Check sheet for the modelled part. Datum: model origin and axes. Units: mm. Round coordinates to 2 decimals unless told otherwise and drop trailing zeros. Loops run counter-clockwise (first coordinate to the right, second up) from the corner with the lowest first, then second, coordinate; pieces in that order, holes last. Notation, with made-up numbers: (-28.5, 29.25) - (27.5, 29.25) arc R16 cw to (27.5, 45.25) - close; hole circle Ø8 at (3, 10). An arc over 180 degrees is marked (long way). Put each result on its own line as item: value.
```python
from build123d import *

# Parameters (mm, degrees)
SKETCH1_W           = 89.5
SKETCH1_H           = 50.8
BOSS_EXTRUDE1_DEPTH = 1.5875
CHAMFER1_SIZE       = 2
SKETCH2_W           = 17.9768
SKETCH2_H           = 11.576
SKETCH2_W_2         = 9.4
SKETCH2_H_2         = 11.4
CUT_EXTRUDE1_DEPTH  = 2.5875
SKETCH3_R           = 1.75
CUT_EXTRUDE2_DEPTH  = 2.5875
CHAMFER2_SIZE       = 1.27
CUT_EXTRUDE3_DEPTH  = 2.5875


with BuildPart() as part:
    # Sketch1 → Boss-Extrude1 (new body)
    with BuildSketch(Plane.XY):
        with Locations((44.75, 25.4)):
            Rectangle(SKETCH1_W, SKETCH1_H)
    extrude(amount=BOSS_EXTRUDE1_DEPTH)

    # Chamfer1
    chamfer1_edges = [part.edges().sort_by_distance(p)[0] for p in [
        (0, 50.8, 0.79375),
        (89.5, 50.8, 0.79375),
        (89.5, 0, 0.79375),
        (0, 0, 0.79375),
    ]]
    chamfer(chamfer1_edges, length=CHAMFER1_SIZE)

    # Sketch2 → Cut-Extrude1 (cut, through all)
    with BuildSketch(Plane.XY.offset(1.5875)):
        with Locations((37.701291048, 34.400499876)):
            Rectangle(SKETCH2_W, SKETCH2_H)
        with Locations((62.186773048, 34.312499876)):
            Rectangle(SKETCH2_W_2, SKETCH2_H_2)
        with BuildLine():
            Line((55.722947048, 29.966053267), (55.722947048, 30.712499876))
            ThreePointArc((55.722947048, 30.712499876), (55.503277134, 31.242829962), (54.972947048, 31.462499876))
            Line((54.972947048, 31.462499876), (48.572947048, 31.462499876))
            ThreePointArc((48.572947048, 31.462499876), (48.042616962, 31.242829962), (47.822947048, 30.712499876))
            Line((47.822947048, 30.712499876), (47.822947048, 29.966053267))
            ThreePointArc((47.822947048, 29.966053267), (47.880037399, 29.679040693), (48.042616962, 29.435723181))
            Line((48.042616962, 29.435723181), (48.646170353, 28.83216979))
            ThreePointArc((48.646170353, 28.83216979), (48.889487865, 28.669590227), (49.176500439, 28.612499876))
            Line((49.176500439, 28.612499876), (54.369393658, 28.612499876))
            ThreePointArc((54.369393658, 28.612499876), (54.656406232, 28.669590227), (54.899723744, 28.83216979))
            Line((54.899723744, 28.83216979), (55.503277134, 29.435723181))
            ThreePointArc((55.503277134, 29.435723181), (55.665856698, 29.679040693), (55.722947048, 29.966053267))
        make_face()
    extrude(amount=-CUT_EXTRUDE1_DEPTH, mode=Mode.SUBTRACT)

    # Sketch3 → Cut-Extrude2 (cut, through all)
    with BuildSketch(Plane.XY.offset(1.5875)):
        with Locations((3.75, 47.15)):
            Circle(SKETCH3_R)
        with Locations((3.75, 3.65)):
            Circle(SKETCH3_R)
        with Locations((85.75, 3.65)):
            Circle(SKETCH3_R)
        with Locations((85.75, 47.15)):
            Circle(SKETCH3_R)
    extrude(amount=-CUT_EXTRUDE2_DEPTH, mode=Mode.SUBTRACT)

    # Chamfer2
    chamfer2_edges = [part.edges().sort_by_distance(p)[0] for p in [
        (2, 47.15, 1.5875),
        (2, 3.65, 1.5875),
        (84, 3.65, 1.5875),
        (84, 47.15, 1.5875),
    ]]
    chamfer(chamfer2_edges, length=CHAMFER2_SIZE)

    # Sketch4 → Cut-Extrude3 (cut, through all)
    with BuildSketch(Plane.XY.offset(1.5875)):
        with BuildLine():
            Line((71.340625, 46.99), (71.340625, 3.81))
            ThreePointArc((71.340625, 3.81), (70.15, 2.619375), (68.959375, 3.81))
            Line((68.959375, 3.81), (68.959375, 46.99))
            ThreePointArc((68.959375, 46.99), (70.15, 48.180625), (71.340625, 46.99))
        make_face()
        with BuildLine():
            Line((45.940625, 46.99), (45.940625, 43.998499876))
            ThreePointArc((45.940625, 43.998499876), (44.75, 42.807874876), (43.559375, 43.998499876))
            Line((43.559375, 43.998499876), (43.559375, 46.99))
            ThreePointArc((43.559375, 46.99), (44.75, 48.180625), (45.940625, 46.99))
        make_face()
        with BuildLine():
            Line((45.940625, 24.802499876), (45.940625, 3.81))
            ThreePointArc((45.940625, 3.81), (44.75, 2.619375), (43.559375, 3.81))
            Line((43.559375, 3.81), (43.559375, 24.802499876))
            ThreePointArc((43.559375, 24.802499876), (44.75, 25.993124876), (45.940625, 24.802499876))
        make_face()
        with BuildLine():
            Line((51.020625, 46.99), (51.020625, 43.998499876))
            ThreePointArc((51.020625, 43.998499876), (49.83, 42.807874876), (48.639375, 43.998499876))
            Line((48.639375, 43.998499876), (48.639375, 46.99))
            ThreePointArc((48.639375, 46.99), (49.83, 48.180625), (51.020625, 46.99))
        make_face()
        with BuildLine():
            Line((51.020625, 24.802499876), (51.020625, 3.81))
            ThreePointArc((51.020625, 3.81), (49.83, 2.619375), (48.639375, 3.81))
            Line((48.639375, 3.81), (48.639375, 24.802499876))
            ThreePointArc((48.639375, 24.802499876), (49.83, 25.993124876), (51.020625, 24.802499876))
        make_face()
        with BuildLine():
            Line((56.100625, 46.99), (56.100625, 43.998499876))
            ThreePointArc((56.100625, 43.998499876), (54.91, 42.807874876), (53.719375, 43.998499876))
            Line((53.719375, 43.998499876), (53.719375, 46.99))
            ThreePointArc((53.719375, 46.99), (54.91, 48.180625), (56.100625, 46.99))
        make_face()
        with BuildLine():
            Line((56.100625, 24.802499876), (56.100625, 3.81))
            ThreePointArc((56.100625, 3.81), (54.91, 2.619375), (53.719375, 3.81))
            Line((53.719375, 3.81), (53.719375, 24.802499876))
            ThreePointArc((53.719375, 24.802499876), (54.91, 25.993124876), (56.100625, 24.802499876))
        make_face()
        with BuildLine():
            Line((61.180625, 46.99), (61.180625, 43.998499876))
            ThreePointArc((61.180625, 43.998499876), (59.99, 42.807874876), (58.799375, 43.998499876))
            Line((58.799375, 43.998499876), (58.799375, 46.99))
            ThreePointArc((58.799375, 46.99), (59.99, 48.180625), (61.180625, 46.99))
        make_face()
        with BuildLine():
            Line((61.180625, 24.802499876), (61.180625, 3.81))
            ThreePointArc((61.180625, 3.81), (59.99, 2.619375), (58.799375, 3.81))
            Line((58.799375, 3.81), (58.799375, 24.802499876))
            ThreePointArc((58.799375, 24.802499876), (59.99, 25.993124876), (61.180625, 24.802499876))
        make_face()
        with BuildLine():
            Line((66.260625, 46.99), (66.260625, 43.998499876))
            ThreePointArc((66.260625, 43.998499876), (65.07, 42.807874876), (63.879375, 43.998499876))
            Line((63.879375, 43.998499876), (63.879375, 46.99))
            ThreePointArc((63.879375, 46.99), (65.07, 48.180625), (66.260625, 46.99))
        make_face()
        with BuildLine():
            Line((66.260625, 24.802499876), (66.260625, 3.81))
            ThreePointArc((66.260625, 3.81), (65.07, 2.619375), (63.879375, 3.81))
            Line((63.879375, 3.81), (63.879375, 24.802499876))
            ThreePointArc((63.879375, 24.802499876), (65.07, 25.993124876), (66.260625, 24.802499876))
        make_face()
        with BuildLine():
            Line((76.420625, 46.99), (76.420625, 3.81))
            ThreePointArc((76.420625, 3.81), (75.23, 2.619375), (74.039375, 3.81))
            Line((74.039375, 3.81), (74.039375, 46.99))
            ThreePointArc((74.039375, 46.99), (75.23, 48.180625), (76.420625, 46.99))
        make_face()
        with BuildLine():
            Line((81.500625, 46.99), (81.500625, 3.81))
            ThreePointArc((81.500625, 3.81), (80.31, 2.619375), (79.119375, 3.81))
            Line((79.119375, 3.81), (79.119375, 46.99))
            ThreePointArc((79.119375, 46.99), (80.31, 48.180625), (81.500625, 46.99))
        make_face()
        with BuildLine():
            Line((7.999375, 46.99), (7.999375, 3.81))
            ThreePointArc((7.999375, 3.81), (9.19, 2.619375), (10.380625, 3.81))
            Line((10.380625, 3.81), (10.380625, 46.99))
            ThreePointArc((10.380625, 46.99), (9.19, 48.180625), (7.999375, 46.99))
        make_face()
        with BuildLine():
            Line((13.079375, 46.99), (13.079375, 3.81))
            ThreePointArc((13.079375, 3.81), (14.27, 2.619375), (15.460625, 3.81))
            Line((15.460625, 3.81), (15.460625, 46.99))
            ThreePointArc((15.460625, 46.99), (14.27, 48.180625), (13.079375, 46.99))
        make_face()
        with BuildLine():
            Line((18.159375, 46.99), (18.159375, 3.81))
            ThreePointArc((18.159375, 3.81), (19.35, 2.619375), (20.540625, 3.81))
            Line((20.540625, 3.81), (20.540625, 46.99))
            ThreePointArc((20.540625, 46.99), (19.35, 48.180625), (18.159375, 46.99))
        make_face()
        with BuildLine():
            Line((23.239375, 46.99), (23.239375, 3.81))
            ThreePointArc((23.239375, 3.81), (24.43, 2.619375), (25.620625, 3.81))
            Line((25.620625, 3.81), (25.620625, 46.99))
            ThreePointArc((25.620625, 46.99), (24.43, 48.180625), (23.239375, 46.99))
        make_face()
        with BuildLine():
            Line((28.319375, 24.802499876), (28.319375, 3.81))
            ThreePointArc((28.319375, 3.81), (29.51, 2.619375), (30.700625, 3.81))
            Line((30.700625, 3.81), (30.700625, 24.802499876))
            ThreePointArc((30.700625, 24.802499876), (29.51, 25.993124876), (28.319375, 24.802499876))
        make_face()
        with BuildLine():
            Line((28.319375, 46.99), (28.319375, 43.998499876))
            ThreePointArc((28.319375, 43.998499876), (29.51, 42.807874876), (30.700625, 43.998499876))
            Line((30.700625, 43.998499876), (30.700625, 46.99))
            ThreePointArc((30.700625, 46.99), (29.51, 48.180625), (28.319375, 46.99))
        make_face()
        with BuildLine():
            Line((33.399375, 24.802499876), (33.399375, 3.81))
            ThreePointArc((33.399375, 3.81), (34.59, 2.619375), (35.780625, 3.81))
            Line((35.780625, 3.81), (35.780625, 24.802499876))
            ThreePointArc((35.780625, 24.802499876), (34.59, 25.993124876), (33.399375, 24.802499876))
        make_face()
        with BuildLine():
            Line((33.399375, 46.99), (33.399375, 43.998499876))
            ThreePointArc((33.399375, 43.998499876), (34.59, 42.807874876), (35.780625, 43.998499876))
            Line((35.780625, 43.998499876), (35.780625, 46.99))
            ThreePointArc((35.780625, 46.99), (34.59, 48.180625), (33.399375, 46.99))
        make_face()
        with BuildLine():
            Line((38.479375, 24.802499876), (38.479375, 3.81))
            ThreePointArc((38.479375, 3.81), (39.67, 2.619375), (40.860625, 3.81))
            Line((40.860625, 3.81), (40.860625, 24.802499876))
            ThreePointArc((40.860625, 24.802499876), (39.67, 25.993124876), (38.479375, 24.802499876))
        make_face()
        with BuildLine():
            Line((38.479375, 46.99), (38.479375, 43.998499876))
            ThreePointArc((38.479375, 43.998499876), (39.67, 42.807874876), (40.860625, 43.998499876))
            Line((40.860625, 43.998499876), (40.860625, 46.99))
            ThreePointArc((40.860625, 46.99), (39.67, 48.180625), (38.479375, 46.99))
        make_face()
    extrude(amount=-CUT_EXTRUDE3_DEPTH, mode=Mode.SUBTRACT)


solid = part.part
```
Item 1: Section check A-A on x = 3.75. Enter the section's corners in (y, z), then the cut area to 3 significant figures.
Filled sheet:
outline: (0, 0) - (1.9, 0) - (1.9, 0.32) - (0.63, 1.59) - (0, 1.59) - close; (5.4, 0) - (45.4, 0) - (45.4, 0.32) - (44.13, 1.59) - (6.67, 1.59) - (5.4, 0.32) - close; (48.9, 0) - (50.8, 0) - (50.8, 1.59) - (50.17, 1.59) - (48.9, 0.32) - close
area: 66.3 mm²
Item 2: Thickness scan on line 1 (Y direction, x = 85.75, z = 0.2); line 2 (Y direction, x = 53.5, z = 1.1); line 3 (Y direction, x = 15, z = 0.45). Record the ranges inside material, lowest first. Write a range as from..to.
Filled sheet:
line 1: 0..1.9, 5.4..45.4, 48.9..50.8
line 2: 0..28.61, 31.46..50.8
line 3: 0..2.87, 47.93..50.8
Item 3: Section check D-D on x = 59.99. Enter the section's corners in (y, z).
Filled sheet:
outline: (0, 0) - (2.62, 0) - (2.62, 1.59) - (0, 1.59) - close; (25.99, 0) - (28.61, 0) - (28.61, 1.59) - (25.99, 1.59) - close; (40.01, 0) - (42.81, 0) - (42.81, 1.59) - (40.01, 1.59) - close; (48.18, 0) - (50.8, 0) - (50.8, 1.59) - (48.18, 1.59) - close
Item 4: Release check for a two-part mould opening along X. For faces 1 (the flat face through (54, 26, 1.588)), 2 (the flat face through (76.421, 26, 1)) record: +X half, -X half, draft (parallel to the pull), parting line (faces both ways), or undercut.
Filled sheet:
face 1: draft
face 2: undercut
Item 5: Section check B-B on x = 75.23. Enter the section's corners in (y, z).
Filled sheet:
outline: (0, 0) - (2.62, 0) - (2.62, 1.59) - (0, 1.59) - close; (48.18, 0) - (50.8, 0) - (50.8, 1.59) - (48.18, 1.59) - close
Item 6: Section check C-C on y = 22. Count the separate pieces of the cut face and the enclosed holes in it, then the cut area to 3 significant figures.
Filled sheet:
separate pieces: 16
enclosed holes: 0
area: 85.4 mm²
